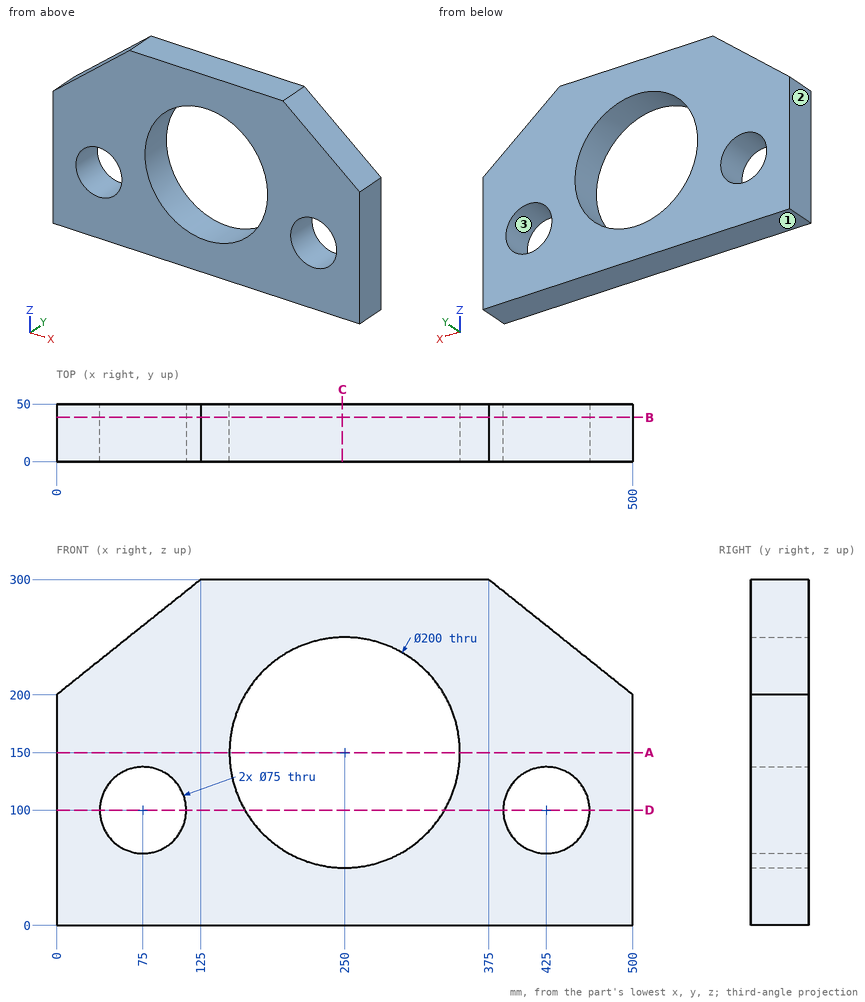
Design review of the part shown in the three views and the two pictorial views. Dimensions are in mm from the part's minimum x, y and z. Round coordinates to 2 decimals unless told otherwise and drop trailing zeros. Order: outer loops, then holes, each group sorted by start corner. A loop starts at its lowest first (then second) coordinate and runs counter-clockwise, first axis right, second up.
Item 1: Add section C-C, the plane x = 248. State the section outline as (y, z) points, and give its area (3 significant figures).
Working result:
outline: (0, 0) - (50, 0) - (50, 50.02) - (0, 50.02) - close; (0, 249.98) - (50, 249.98) - (50, 300) - (0, 300) - close
area: 5,000 mm2
Item 2: Draft analysis for pull direction X (two halves, no side actions). For the marked faces 1, 2 and 3, state which applies: released by +X, released by -X, zero draft, split by the parting line, or undercut.
Working result:
face 1: zero draft
face 2: released by -X
face 3: undercut
Item 3: Add section A-A, the plane z = 150. State the section outline as (x, y) points, and give its area (3 significant figures).
Working result:
outline: (0, 0) - (150, 0) - (150, 50) - (0, 50) - close; (350, 0) - (500, 0) - (500, 50) - (350, 50) - close
area: 15,000 mm2
Item 4: To check wall thickness, follow probe 1 along Z at (x, y) = (250, 33); probe 2 along X at (y, z) = (24, 152); probe 3 along Z at (x, y) = (242.5, 15). State the ranges of each line that lie inside material, in increasing order.
Working result:
probe 1: z = 0 to 50, 250 to 300
probe 2: x = 0 to 150.02, 349.98 to 500
probe 3: z = 0 to 50.28, 249.72 to 300
Item 5: Add section B-B, the plane y = 38.5. State the section outline as (x, z) points.
Working result:
outline: (0, 0) - (500, 0) - (500, 200) - (375, 300) - (125, 300) - (0, 200) - close; hole circle Ø75 at (75, 100); hole circle Ø200 at (250, 150); hole circle Ø75 at (425, 100)
Item 6: Add section D-D, the plane z = 100. State the section outline as (x, y) points, and give its area (3 significant figures).
Working result:
outline: (0, 0) - (37.5, 0) - (37.5, 50) - (0, 50) - close; (112.5, 0) - (163.4, 0) - (163.4, 50) - (112.5, 50) - close; (336.6, 0) - (387.5, 0) - (387.5, 50) - (336.6, 50) - close; (462.5, 0) - (500, 0) - (500, 50) - (462.5, 50) - close
area: 8,840 mm2
Item 7: For pin 1 (6 mm diameter, centred on x = 362, z = 36, fed in from -Y); pin 2 (6 mm diameter, centred on x = 97.5, y = 20.5, fed in from +Z); pin 3 (2 mm diameter, centred on y = 43, z = 253.5, fed in from +X) (3 decimals), all flat-tipped, find the tip position at first contact; note any pin that passes through.
Working result:
pin 1: stops at y = 0
pin 2: stops at z = 280.4
pin 3: stops at x = 434.375
